from build123d import *


with BuildPart() as part:
    # Toroidal Core → Revolve2 (revolve)
    with BuildSketch(Plane.XY, mode=Mode.PRIVATE) as revolve2_sk:
        with BuildLine():
            Line((11.59739394, 0), (18.713632535, 0))
            ThreePointArc((18.713632535, 0), (18.816911461, 0.042779532), (18.859690994, 0.146058459))
            Line((18.859690994, 0.146058459), (18.859690994, 10.640147279))
            ThreePointArc((18.859690994, 10.640147279), (18.816911461, 10.743426205), (18.713632535, 10.786205737))
            Line((18.713632535, 10.786205737), (11.59739394, 10.786205737))
            ThreePointArc((11.59739394, 10.786205737), (11.494115013, 10.743426205), (11.451335481, 10.640147279))
            Line((11.451335481, 10.640147279), (11.451335481, 0.146058459))
            ThreePointArc((11.451335481, 0.146058459), (11.494115013, 0.042779532), (11.59739394, 0))
        make_face()
    revolve(revolve2_sk.sketch.rotate(Axis((0, -8.107972275, 0), (0, 1, 0)), 90), axis=Axis((0, -8.107972275, 0), (0, 1, 0)))


solid = part.part
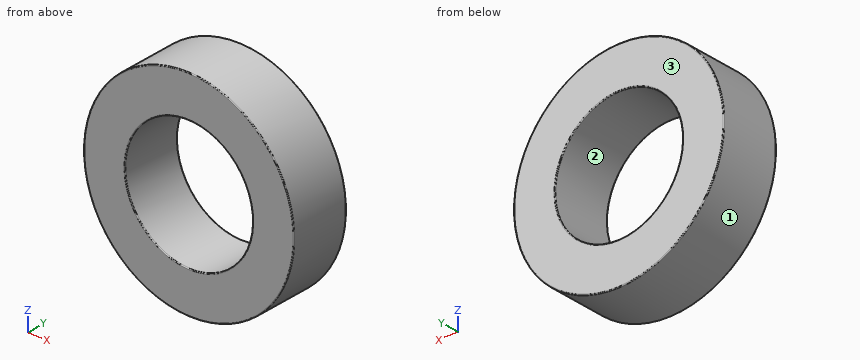
Geometry check sheet. Reference: the model listing, model coordinates, mm. Face numbers are marked on the shaded views. Give positions to 0.01 mm unless a question says otherwise; leave off trailing zeros. Loops run counter-clockwise (first coordinate to the right, second up) from the corner with the lowest first, then second, coordinate; pieces in that order, holes last. Notation, with made-up numbers: (50, 56) -> (86, 56) arc R8 ccw to (86, 62) -> close; hole circle Ø4 at (38, -28.5). An arc over 180 degrees is marked (long way). Answer in a Markdown table with one row per item. Add a question column.
1) Cross-section at A-A on z = 0. Record the boundary of the cut face in (x, y).
2) Draft check along X on the marked faces 1, 2 and 3. Enter one of: pulls with the +X half, pulls with the -X half, needs draft (parallel to the pull), parting line crosses it, or undercut.
3) Material ranges on probe 1 along X at (y, z) = (4.75, 0); probe 2 along Z at (x, y) = (8, 10); probe 3 along X at (y, z) = (4, 2.5), recorded low to high. Write a range as from..to.
4) Cross-section at C-C on y = 1. Record the boundary of the cut face in (x, z).
5) Cross-section at B-B on x = 0. Record the boundary of the cut face in (y, z).
6) Gauge pin test, flat ends, axial feed: P1, Ø6, axis at x = -3, z = 12, coming from the -Y side; P2, Ø2, axis at x = -11, y = 9.5, coming from the -Z side; P3, Ø2, axis at y = 6.5, z = 13, coming from the +X side; P4, Ø1.5, axis at y = 2.5, z = -14, coming from the +X side. Record the tip position at first contact, or that the pin passes through.
Outcome:
| question | item | result |
|---|---|---|
| 1 | outline | (-18.86, 0.15) arc R0.15 ccw to (-18.71, 0) -> (-11.6, 0) arc R0.15 ccw to (-11.45, 0.15) -> (-11.45, 10.64) arc R0.15 ccw to (-11.6, 10.79) -> (-18.71, 10.79) arc R0.15 ccw to (-18.86, 10.64) -> close; (11.45, 0.15) arc R0.15 ccw to (11.6, 0) -> (18.71, 0) arc R0.15 ccw to (18.86, 0.15) -> (18.86, 10.64) arc R0.15 ccw to (18.71, 10.79) -> (11.6, 10.79) arc R0.15 ccw to (11.45, 10.64) -> close |
| 2 | face 1 | parting line crosses it |
| 2 | face 2 | undercut |
| 2 | face 3 | needs draft |
| 3 | probe 1 | x = -18.86..-11.45, 11.45..18.86 |
| 3 | probe 2 | z = -17.08..-8.19, 8.19..17.08 |
| 3 | probe 3 | x = -18.69..-11.18, 11.18..18.69 |
| 4 | outline | circle Ø37.72 at (0, 0); hole circle Ø22.9 at (0, 0) |
| 5 | outline | (0, -18.71) arc R0.15 ccw to (0.15, -18.86) -> (10.64, -18.86) arc R0.15 ccw to (10.79, -18.71) -> (10.79, -11.6) arc R0.15 ccw to (10.64, -11.45) -> (0.15, -11.45) arc R0.15 ccw to (0, -11.6) -> close; (0, 11.6) arc R0.15 ccw to (0.15, 11.45) -> (10.64, 11.45) arc R0.15 ccw to (10.79, 11.6) -> (10.79, 18.71) arc R0.15 ccw to (10.64, 18.86) -> (0.15, 18.86) arc R0.15 ccw to (0, 18.71) -> close |
| 6 | P1 | stops at y = 0 |
| 6 | P2 | stops at z = -15.99 |
| 6 | P3 | stops at x = 14.55 |
| 6 | P4 | stops at x = 13.42 |
